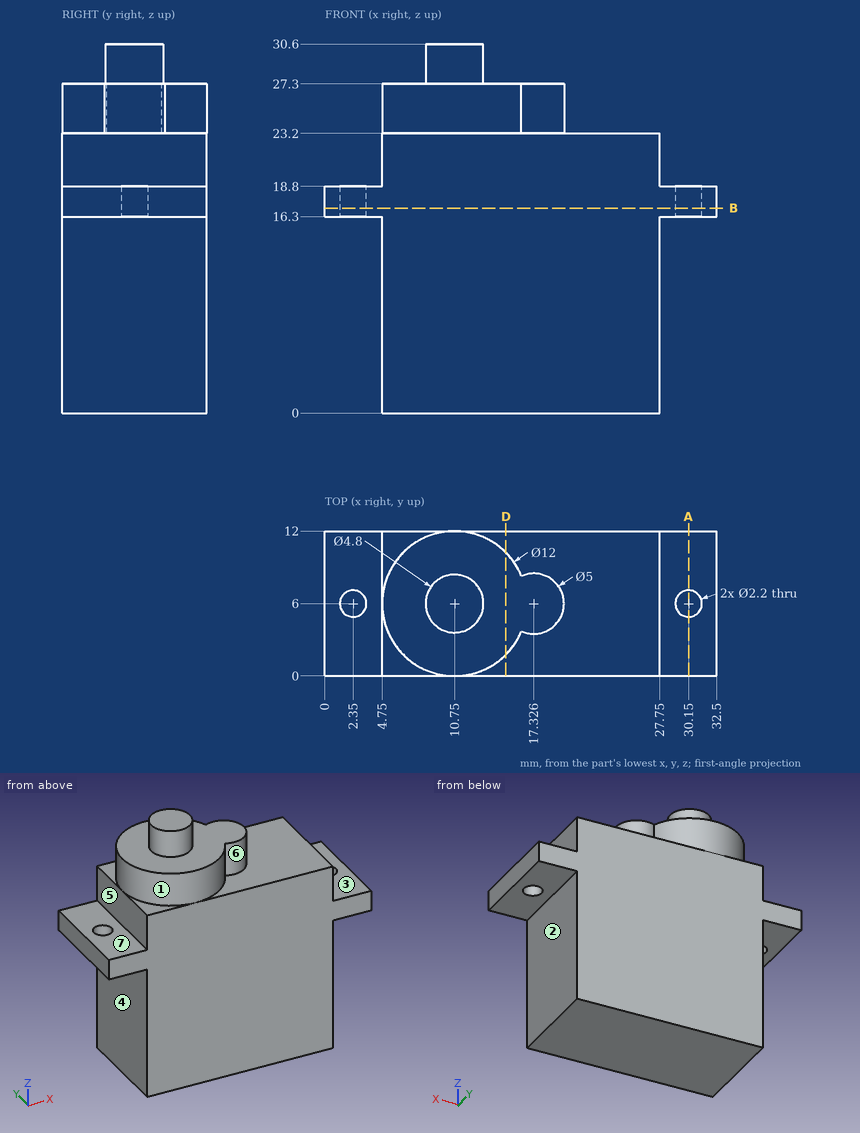
Input: dimensioned drawing with shaded views. Units: mm. Origin: part minimum x, y, z. A direction names the side the tool comes from. Coordinates: 2 decimals unless noted, no trailing zeros. Order: outer loops, then holes, each group sorted by start corner. A loop starts at its lowest first (then second) coordinate and runs counter-clockwise, first axis right, second up.
1. Ray query, line 1 along Y through (x, z) = (30.15, 18.35); line 2 along X through (y, z) = (2.5, 13); line 3 along Z through (x, y) = (25, 7.5). Return the intervals inside material, ascending.
Checked values:
line 1: y = 0 to 4.9, 7.1 to 12
line 2: x = 4.75 to 27.75
line 3: z = 0 to 23.2
2. Cut plane D-D, the plane x = 15. Return loops of the section in (y, z) (1 decimal).
Checked values:
outline: (0, 0) - (12, 0) - (12, 23.2) - (10.2, 23.2) - (10.2, 27.3) - (1.8, 27.3) - (1.8, 23.2) - (0, 23.2) - close
3. Contact query for flat-ended pins moving along their axis: P1, Ø1, axis at y = 10, z = 15, coming from the +X side; P2, Ø1.4, axis at x = 2.5, y = 4, coming from the -Z side; P3, Ø4, axis at x = 31, y = 6.5, coming from the +Z side. Output: stop coordinate, or through.
Checked values:
P1: stops at x = 27.75
P2: stops at z = 16.3
P3: stops at z = 18.8
4. Cut plane B-B, the plane z = 17. Return loops of the section in (x, y).
Checked values:
outline: (0, 0) - (32.5, 0) - (32.5, 12) - (0, 12) - close; hole circle Ø2.2 at (2.35, 6); hole circle Ø2.2 at (30.15, 6)
5. Draft query along X for the marked faces 5, 6 and 7. Return one class per face: +X half, -X half, draft (parallel to the pull), parting line (faces both ways), or undercut.
Checked values:
face 5: -X half
face 6: undercut
face 7: draft
6. Access query for the marked faces 1, 2, 3 and 4. Directions: +Z, -Z, +X, -X, +Y, -Y. A direction counts if a zero-diameter tool reaches every point of the face in a straight line with its end or side. Return the directions, or none.
Checked values:
face 1: +Z
face 2: -Z, +X, +Y, -Y
face 3: +Z, +X, +Y, -Y
face 4: -Z, -X, +Y, -Y
7. Cut plane A-A, the plane x = 30.15. Return loops of the section in (y, z).
Checked values:
outline: (0, 16.3) - (4.9, 16.3) - (4.9, 18.8) - (0, 18.8) - close; (7.1, 16.3) - (12, 16.3) - (12, 18.8) - (7.1, 18.8) - close
